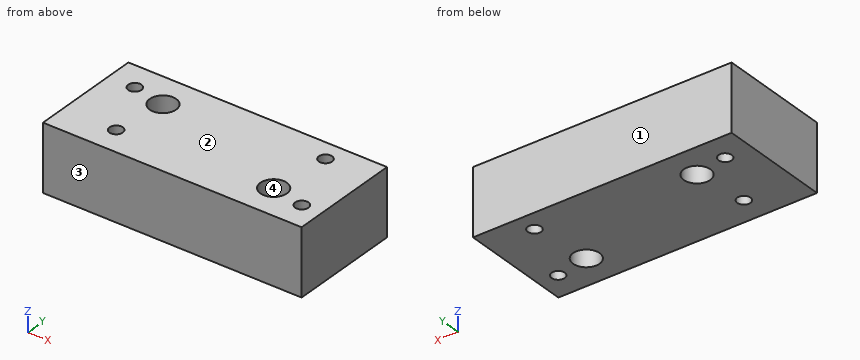
```python
from build123d import *

# Parameters (mm, degrees)
SKETCH1_W           = 39
SKETCH1_H           = 17
SKETCH1_R           = 2
SKETCH1_R_2         = 1
BOSS_EXTRUDE1_DEPTH = 5


with BuildPart() as part:
    # Sketch1 → Boss-Extrude1 (new, symmetric)
    with BuildSketch(Plane.XY):
        Rectangle(SKETCH1_W, SKETCH1_H)
        with Locations((-10.5, 3.5)):
            Circle(SKETCH1_R, mode=Mode.SUBTRACT)
        with Locations((-15.5, 4.5)):
            Circle(SKETCH1_R_2, mode=Mode.SUBTRACT)
        with Locations((-11.5, -4.5)):
            Circle(SKETCH1_R_2, mode=Mode.SUBTRACT)
        with Locations((11.5, -3.5)):
            Circle(SKETCH1_R, mode=Mode.SUBTRACT)
        with Locations((12.5, 5.5)):
            Circle(SKETCH1_R_2, mode=Mode.SUBTRACT)
        with Locations((16.5, -4.5)):
            Circle(SKETCH1_R_2, mode=Mode.SUBTRACT)
    extrude(amount=BOSS_EXTRUDE1_DEPTH, both=True)


solid = part.part
```
Model file for the job. Use its own axes, mm. Face numbers are marked on the shaded views. Coordinates: 2 decimals unless noted, no trailing zeros. Write each loop counter-clockwise with the first axis right and the second up, starting at its lowest first coordinate (ties: lowest second). Pieces come first, ordered by that corner, then holes. Notation, with made-up numbers: (-19.75, 47.25) - (24.25, 47.25) arc R27 ccw to (24.25, 73.25) - close; hole circle Ø6 at (-35, 61.5). An arc over 180 degrees is marked (long way). Use a Markdown table: item, result. Add a question column.
Item 1: Drill centre lines: line 1 along Y through (x, z) = (-15.5, -2); line 2 along Y through (x, z) = (16.5, -3); line 3 along X through (y, z) = (3.75, 3). Where is each one in solid material? Low to high.
Item 2: Band-saw the part on B-B, the plane x = 16.5. Write the cut outline in (y, z), and give its area (3 significant figures).
Item 3: Two-plate mould, pull along Y, no slides. Class the marked faces 1, 2, 3 and 4: pulls with the +Y half, pulls with the -Y half, needs draft (parallel to the pull), parting line crosses it, or undercut.
Item 4: Band-saw the part on C-C, the plane x = 12. Write the cut outline in (y, z).
Item 5: Band-saw the part on A-A, the plane z = 0.25. Write the cut outline in (x, y), and give its area (3 significant figures).
A:
| question | item | result |
|---|---|---|
| 1 | line 1 | y = -8.5 to 3.5, 5.5 to 8.5 |
| 1 | line 2 | y = -8.5 to -5.5, -3.5 to 8.5 |
| 1 | line 3 | x = -19.5 to -16.16, -14.84 to -12.48, -8.52 to 19.5 |
| 2 | outline | (-8.5, -5) - (-5.5, -5) - (-5.5, 5) - (-8.5, 5) - close; (-3.5, -5) - (8.5, -5) - (8.5, 5) - (-3.5, 5) - close |
| 2 | area | 150 mm² |
| 3 | face 1 | pulls with the +Y half |
| 3 | face 2 | needs draft |
| 3 | face 3 | pulls with the -Y half |
| 3 | face 4 | undercut |
| 4 | outline | (-8.5, -5) - (-5.44, -5) - (-5.44, 5) - (-8.5, 5) - close; (-1.56, -5) - (4.63, -5) - (4.63, 5) - (-1.56, 5) - close; (6.37, -5) - (8.5, -5) - (8.5, 5) - (6.37, 5) - close |
| 5 | outline | (-19.5, -8.5) - (19.5, -8.5) - (19.5, 8.5) - (-19.5, 8.5) - close; hole circle Ø2 at (-15.5, 4.5); hole circle Ø2 at (-11.5, -4.5); hole circle Ø4 at (-10.5, 3.5); hole circle Ø4 at (11.5, -3.5); hole circle Ø2 at (12.5, 5.5); hole circle Ø2 at (16.5, -4.5) |
| 5 | area | 625 mm² |
